Input: part model. Units: mm. Frame: model coordinates. Coordinates: 2 decimals unless noted, no trailing zeros. Loops run counter-clockwise (first coordinate to the right, second up) from the corner with the lowest first, then second, coordinate; pieces in that order, holes last.
Item 1: Section B-B on z = 19. Return loops of the section in (x, y).
Item 2: Contact query for flat-ended pins moving along their axis: P1, Ø1.8, axis at x = -9.67, z = -17.22, coming from the +Y side; P2, Ø1, axis at x = 38, y = 1.5, coming from the +Z side. Output: stop coordinate, or through.
Item 3: Section A-A on x = 35. Return loops of the section in (y, z).
Item 4: Section D-D on z = -5.1. Return loops of the section in (x, y).
Item 5: Section C-C on y = 1.05. Give the number of separate pieces and of enclosed holes in the cut face, and give its area (3 significant figures).
Item 6: Ray query, line 1 along X through (y, z) = (0.8, 0); line 2 along Z through (x, y) = (27, 2.2); line 3 along X through (y, z) = (1, -7). Return the intervals inside material, ascending.
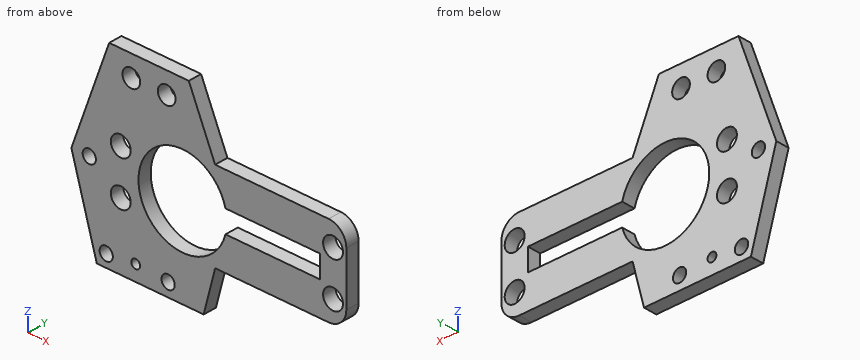
```python
from build123d import *

# Parameters (mm, degrees)
SKETCH_1_R      = 2
SKETCH_1_R_2    = 1
SKETCH_1_R_3    = 1.5
SKETCH_1_R_4    = 2.25
EXTRUDE_1_DEPTH = 3
FILLET_1_R      = 4


with BuildPart() as part:
    # 草图1 → 凸台-拉伸1 (new body)
    with BuildSketch(Plane(origin=(0, 0, 0), x_dir=(1, 0, 0), z_dir=(0, 1, 0))):
        Polygon((-9, -23.780312322), (-17.547496939, 0), (-11.800187967, 20), (12.367390868, 20), (14.956440464, 10), (44.617690385, 10), (44.617690385, -10), (14.956440464, -10), (9, -23.780312322), align=None)
        with Locations(Location((-4, -19, 0), (0, 0, 270))):
            Circle(SKETCH_1_R, mode=Mode.SUBTRACT)
        with Locations(Location((4, -19, 0), (0, 0, 270))):
            Circle(SKETCH_1_R, mode=Mode.SUBTRACT)
        with Locations(Location((-3, 16.5, 0), (0, 0, 270))):
            Circle(SKETCH_1_R_2, mode=Mode.SUBTRACT)
        with Locations(Location((4.324928848, 17, 0), (0, 0, 270))):
            Circle(SKETCH_1_R_3, mode=Mode.SUBTRACT)
        with Locations(Location((41.617690385, 5.1, 0), (0, 0, 270))):
            Circle(SKETCH_1_R_4, mode=Mode.SUBTRACT)
        with Locations(Location((41.617690385, -4.9, 0), (0, 0, 270))):
            Circle(SKETCH_1_R_4, mode=Mode.SUBTRACT)
        with Locations(Location((-6.382309615, -4.9, 0), (0, 0, 270))):
            Circle(SKETCH_1_R_4, mode=Mode.SUBTRACT)
        with Locations(Location((-6.382309615, 5.1, 0), (0, 0, 270))):
            Circle(SKETCH_1_R_4, mode=Mode.SUBTRACT)
        with Locations(Location((-13.5, 0, 0), (0, 0, 270))):
            Circle(SKETCH_1_R_3, mode=Mode.SUBTRACT)
        with Locations(Location((-9.67339824, 17.216422607, 0), (0, 0, 270))):
            Circle(SKETCH_1_R_3, mode=Mode.SUBTRACT)
        with BuildLine():
            Line((17.30014875, -2.5), (38.617690385, -2.5))
            Line((38.617690385, -2.5), (38.617690385, 2.5))
            Line((38.617690385, 2.5), (17.30014875, 2.5))
            ThreePointArc((17.30014875, 2.5), (-2.382309615, 0), (17.30014875, -2.5))
        make_face(mode=Mode.SUBTRACT)
    extrude(amount=EXTRUDE_1_DEPTH)

    # 圆角1
    fillet_1_edges = [part.edges().sort_by_distance(p)[0] for p in [
        (44.617690385, 1.5, -10),
        (44.617690385, 1.5, 10),
    ]]
    fillet(fillet_1_edges, radius=FILLET_1_R)


solid = part.part
```
Results found:
1. outline: (-10.72, 0) - (-6, 0) - (-6, 3) - (-10.72, 3) - close; (-2, 0) - (2, 0) - (2, 3) - (-2, 3) - close; (6, 0) - (11.07, 0) - (11.07, 3) - (6, 3) - close
2. P1: passes through
2. P2: stops at z = 10
3. outline: (0, -10) - (3, -10) - (3, -2.5) - (0, -2.5) - close; (0, 2.5) - (3, 2.5) - (3, 10) - (0, 10) - close
4. outline: (-16.08, 0) - (-8.63, 0) - (-8.63, 3) - (-16.08, 3) - close; (-4.13, 0) - (-0.98, 0) - (-0.98, 3) - (-4.13, 3) - close; (16.22, 0) - (39.37, 0) - (39.37, 3) - (16.22, 3) - close; (43.87, 0) - (44.62, 0) - (44.62, 3) - (43.87, 3) - close
5. separate pieces: 1
5. enclosed holes: 11
5. area: 1,260 mm2
6. line 1: x = -17.55 to -15, -12 to -2.38, 38.62 to 44.62
6. line 2: z = -10 to -2.5, 2.5 to 10
6. line 3: x = -15.54 to -7.59, -5.18 to 0.48, 14.76 to 40.41, 42.82 to 44.49
